```python
from build123d import *

# Parameters (mm, degrees)
F0_W     = 0.79375
F0_H     = 18.25625
F2_R     = 3.175
F2_R_2   = 1.190625
F3_DEPTH = 0.79375


with BuildPart() as f1:
    # F0 (on Right) → F1 (revolve)
    with BuildSketch(Plane.YZ):
        with Locations((-117.871875, 9.128125)):
            Rectangle(F0_W, F0_H)
    revolve(axis=Axis((0, -58.7375, 0), (0, -1, 0)))

    # F2 (on face) → F3 (cut, through all)
    with BuildSketch(Plane.XZ.offset(118.26875)):
        Circle(F2_R)
        with Locations((-7.9375, 0)):
            Circle(F2_R_2)
        with Locations((-6.080478, -5.102127)):
            Circle(F2_R_2)
        with Locations((-1.378332, -7.816912)):
            Circle(F2_R_2)
        with Locations((3.96875, -6.874077)):
            Circle(F2_R_2)
        with Locations((7.45881, -2.714785)):
            Circle(F2_R_2)
        with Locations((7.45881, 2.714785)):
            Circle(F2_R_2)
        with Locations((3.96875, 6.874077)):
            Circle(F2_R_2)
        with Locations((-1.378332, 7.816912)):
            Circle(F2_R_2)
        with Locations((-6.080478, 5.102127)):
            Circle(F2_R_2)
    extrude(amount=-F3_DEPTH, mode=Mode.SUBTRACT)


solid = f1.part
```
Model file for the job. Use its own axes, mm. Coordinates: 2 decimals unless noted, no trailing zeros. Loops run counter-clockwise (first coordinate to the right, second up) from the corner with the lowest first, then second, coordinate; pieces in that order, holes last. Notation, with made-up numbers: (-31.5, 26.5) - (23.5, 26.5) arc R26 ccw to (23.5, 50.5) - close; hole circle Ø3 at (22.25, 17.5). An arc over 180 degrees is marked (long way). Answer as a JSON object with one key per item and string values. Group by question number.
(1) Cut at A-A (z = 0). Give the cut face in (x, y) (3 decimals).
(2) Probe line 1 along Z through (x, y) = (3.5, -117.9); line 2 along Z through (x, y) = (6.5, -117.7); line 3 along Z through (x, y) = (0, -117.85) (3 decimals). List the from-to ranges inside material, lowest first.
(3) Cut at D-D (z = 4.5). Give the cut face in (x, y) (3 decimals).
(4) Cut at B-B (x = 4.5). Give the cut face in (y, z) (3 decimals), then the cut area to 3 significant figures.
(5) Two-plate mould, pull along X, no slides. Class faces 1 (the face through (2.78, -117.88, 6.93)), 2 (the face through (-5.484, -117.866, 17.413)), 3 (the face through (4, -117.475, 0)): released by +X, released by -X, zero draft, split by the parting line, or undercut.
(6) Cut at C-C (y = -118.1). State how many separate pieces and enclosed holes the cut face has, then the cut area to 3 significant figures.
Geometry says:
{
 "1": {"outline": "(-18.256, -118.269) - (-9.128, -118.269) - (-9.128, -117.475) - (-18.256, -117.475) - close; (-6.747, -118.269) - (-3.175, -118.269) - (-3.175, -117.475) - (-6.747, -117.475) - close; (3.175, -118.269) - (18.256, -118.269) - (18.256, -117.475) - (3.175, -117.475) - close"},
 "2": {"line 1": "z = -17.92 to -7.97, -5.78 to 5.78, 7.97 to 17.92", "line 2": "z = -17.06 to -3.42, -2.01 to 2.01, 3.42 to 17.06", "line 3": "z = -18.256 to -3.175, 3.175 to 18.256"},
 "3": {"outline": "(-17.693, -118.269) - (-7.108, -118.269) - (-7.108, -117.475) - (-17.693, -117.475) - close; (-5.053, -118.269) - (17.693, -118.269) - (17.693, -117.475) - (-5.053, -117.475) - close"},
 "4": {"outline": "(-118.269, -17.693) - (-117.475, -17.693) - (-117.475, -7.94) - (-118.269, -7.94) - close; (-118.269, -5.809) - (-117.475, -5.809) - (-117.475, 5.809) - (-118.269, 5.809) - close; (-118.269, 7.94) - (-117.475, 7.94) - (-117.475, 17.693) - (-118.269, 17.693) - close", "area": "24.7 mm^2"},
 "5": {"face 1": "undercut", "face 2": "split by the parting line", "face 3": "zero draft"},
 "6": {"separate pieces": "1", "enclosed holes": "10", "area": "975 mm^2"}
}
